from build123d import *

# Parameters (mm, degrees)
IZIM1_R                     = 16.5
IZIM1_R_2                   = 2.5
Y_KSEKLIK_EKSTR_ZYON2_DEPTH = 11.5
IZIM1_4_R                   = 16.5
IZIM1_4_R_2                 = 12.5
Y_KSEKLIK_EKSTR_ZYON4_DEPTH = 12


with BuildPart() as part:
    # izim1 → Y_kseklik-Ekstr_zyon2 (new body)
    with BuildSketch(Plane.XY):
        with BuildLine():
            ThreePointArc((18.33030278, 8), (14.142135624, 14.142135624), (8, 18.33030278))
            ThreePointArc((8, 18.33030278), (5.816699867, 20.174265687), (5, 22.912878475))
            Line((5, 22.912878475), (5, 28.75))
            ThreePointArc((5, 28.75), (0, 33.75), (-5, 28.75))
            Line((-5, 28.75), (-5, 22.912878475))
            ThreePointArc((-5, 22.912878475), (-5.816699867, 20.174265687), (-8, 18.33030278))
            ThreePointArc((-8, 18.33030278), (-14.142135624, 14.142135624), (-18.33030278, 8))
            ThreePointArc((-18.33030278, 8), (-20.174265687, 5.816699867), (-22.912878475, 5))
            Line((-22.912878475, 5), (-28.75, 5))
            ThreePointArc((-28.75, 5), (-33.75, 0), (-28.75, -5))
            Line((-28.75, -5), (-22.912878475, -5))
            ThreePointArc((-22.912878475, -5), (-20.174265687, -5.816699867), (-18.33030278, -8))
            ThreePointArc((-18.33030278, -8), (0, -20), (18.33030278, -8))
            ThreePointArc((18.33030278, -8), (20.174265687, -5.816699867), (22.912878475, -5))
            Line((22.912878475, -5), (28.75, -5))
            ThreePointArc((28.75, -5), (33.75, 0), (28.75, 5))
            Line((28.75, 5), (22.912878475, 5))
            ThreePointArc((22.912878475, 5), (20.174265687, 5.816699867), (18.33030278, 8))
        make_face()
        Circle(IZIM1_R, mode=Mode.SUBTRACT)
        with Locations((0, 28.75)):
            Circle(IZIM1_R_2, mode=Mode.SUBTRACT)
        with Locations((28.75, 0)):
            Circle(IZIM1_R_2, mode=Mode.SUBTRACT)
        with Locations((-28.75, 0)):
            Circle(IZIM1_R_2, mode=Mode.SUBTRACT)
    extrude(amount=Y_KSEKLIK_EKSTR_ZYON2_DEPTH)

    # izim1_4 → Y_kseklik-Ekstr_zyon4 (add)
    with BuildSketch(Plane.XY):
        Circle(IZIM1_4_R)
        Circle(IZIM1_4_R_2, mode=Mode.SUBTRACT)
    extrude(amount=Y_KSEKLIK_EKSTR_ZYON4_DEPTH)


solid = part.part
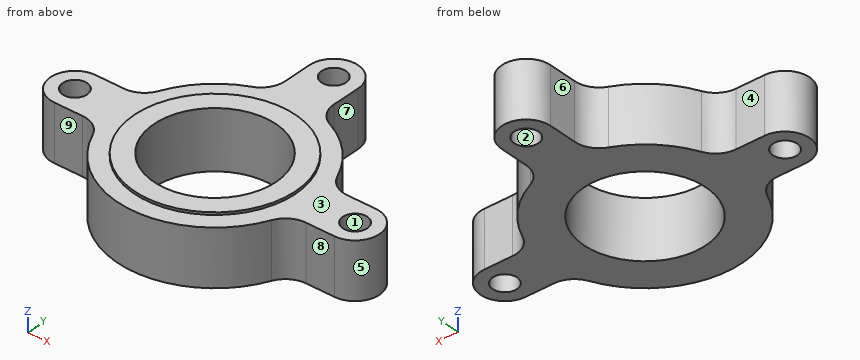
Input: part model. Units: mm. Frame: model coordinates. Face numbers are marked on the shaded views. A direction names the side the tool comes from. Give positions to 0.01 mm unless a question says otherwise; leave off trailing zeros. Loops run counter-clockwise (first coordinate to the right, second up) from the corner with the lowest first, then second, coordinate; pieces in that order, holes last. Notation, with made-up numbers: M -14.5,-24.75 L 22.5,-24.75 A18 ccw 22.5,-18.75 Z; hole C 0.25,-20 d11. An arc over 180 degrees is marked long. Use CSV: the item, a comma, the result in double quotes.
(1) Pin query (flat end, axial travel): P1, Ø4, axis at y = 5, z = 9, coming from the +X side; P2, Ø2, axis at x = 2.5, y = 25.5, coming from the +Z side; P3, Ø3, axis at y = -11.5, z = 4, coming from the -X side; P4, Ø3, axis at x = 4.5, y = -12.5, coming from the -Z side. Return the tip coordinate at first contact, or that it passes through.
Outcome:
P1,"stops at x = 32.75"
P2,"stops at z = 11.5"
P3,"stops at x = -17.32"
P4,"stops at z = 0"
(2) Material intervals for L1, parallel to Y at x = -29, z = 8.75; L2, parallel to X at y = 28.5, z = 1; L3, parallel to X at y = 28, z = 1.25, sorted ascending. Write a range as [from, to].
Outcome:
L1,"y = [-4.99, -2.49], [2.49, 4.99]"
L2,"x = [-5, -2.49], [2.49, 5]"
L3,"x = [-5, -2.38], [2.38, 5]"
(3) Pull-direction query (Y, two-part tool) for the marked faces 1, 2, 3 and 4; classes: pulls with the +Y half, pulls with the -Y half, needs draft (parallel to the pull), parting line crosses it, or undercut.
Outcome:
face 1,"undercut"
face 2,"undercut"
face 3,"needs draft"
face 4,"pulls with the +Y half"
(4) Section D-D, the plane x = 13.5. Return loops of the section in (y, z).
Outcome:
outline,"M -14.76,0 L 14.76,0 L 14.76,11.5 L 9.49,11.5 L 9.49,12 L -9.49,12 L -9.49,11.5 L -14.76,11.5 Z"
(5) Section A-A, the plane z = 8.5. Return loops of the section in (x, y).
Outcome:
outline,"M -28.75,-5 L -22.91,-5 A5 cw -18.33,-8 A20 ccw 18.33,-8 A5 cw 22.91,-5 L 28.75,-5 A5 ccw 28.75,5 L 22.91,5 A5 cw 18.33,8 A20 ccw 8,18.33 A5 cw 5,22.91 L 5,28.75 A5 ccw -5,28.75 L -5,22.91 A5 cw -8,18.33 A20 ccw -18.33,8 A5 cw -22.91,5 L -28.75,5 A5 ccw Z; hole C -28.75,0 d5; hole C 0,0 d25; hole C 0,28.75 d5; hole C 28.75,0 d5"
(6) Set-up query: the marked faces 5, 6, 7, 8 and 9. Return all of +Z, -Z, +X, -X, +Y, -Y with unobstructed straight access to the full face (end or side cutting, diameter ignored); none if empty.
Outcome:
face 5,"+Z, -Z, +X"
face 6,"+Z, -Z, -X, +Y"
face 7,"+Z, -Z, +X, +Y"
face 8,"+Z, -Z, +X, -Y"
face 9,"+Z, -Z, -X, -Y"
(7) Section B-B, the plane x = 0. Return loops of the section in (y, z).
Outcome:
outline,"M -20,0 L -12.5,0 L -12.5,12 L -16.5,12 L -16.5,11.5 L -20,11.5 Z; M 12.5,0 L 26.25,0 L 26.25,11.5 L 16.5,11.5 L 16.5,12 L 12.5,12 Z; M 31.25,0 L 33.75,0 L 33.75,11.5 L 31.25,11.5 Z"
(8) Section C-C, the plane y = 27. Return loops of the section in (x, z).
Outcome:
outline,"M -5,0 L -1.79,0 L -1.79,11.5 L -5,11.5 Z; M 1.79,0 L 5,0 L 5,11.5 L 1.79,11.5 Z"
